from build123d import *

# Parameters (mm, degrees)
SKETCH1_W           = 26
SKETCH1_H           = 10
BOSS_EXTRUDE1_DEPTH = 4


with BuildPart() as part:
    # Sketch1 → Boss-Extrude1 (new body)
    with BuildSketch(Plane.XY):
        with Locations((13, 5)):
            Rectangle(SKETCH1_W, SKETCH1_H)
        Polygon((2.899999851, 6.905256103), (4.382026, 7.166577107), (5.68529807, 6.414133033), (6.200000003, 5.000000051), (5.68529807, 3.585867069), (4.382026, 2.833422995), (2.899999851, 3.094743999), (1.932676008, 4.247555672), (1.932676008, 5.75244443), align=None, mode=Mode.SUBTRACT)
        Polygon((20.899999848, 6.905256103), (22.382025996, 7.166577107), (23.685298066, 6.414133033), (24.2, 5.000000051), (23.685298066, 3.585867069), (22.382025996, 2.833422995), (20.899999848, 3.094743999), (19.932676005, 4.247555672), (19.932676005, 5.75244443), align=None, mode=Mode.SUBTRACT)
    extrude(amount=BOSS_EXTRUDE1_DEPTH)


solid = part.part
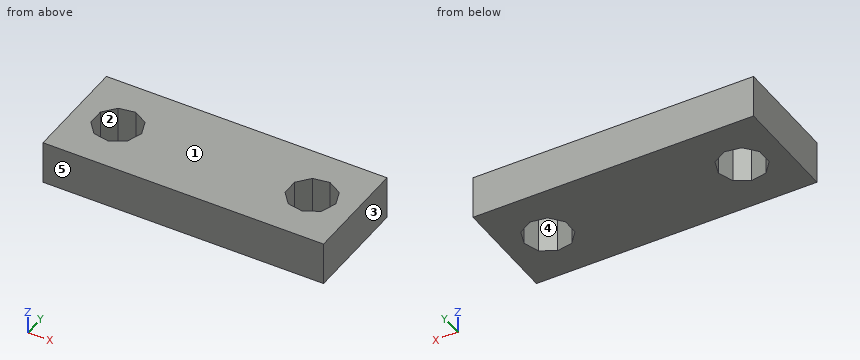
For this review, take the finished solid that the model builds, in its own axes (mm). Face numbers are marked on the shaded views. A direction names the side the tool comes from. Give positions to 0.01 mm unless a question says otherwise; leave off trailing zeros. Loops run counter-clockwise (first coordinate to the right, second up) from the corner with the lowest first, then second, coordinate; pieces in that order, holes last.
Item 1: Take a section at B-B, the plane x = 22.75. State the section outline as (y, z) points.
Item 2: Take a section at A-A, the plane z = 1.25. State the section outline as (x, y) points, and give its area (3 significant figures).
Item 3: Draft analysis for pull direction X (two halves, no side actions). For the marked faces 1, 2 and 3, state which applies: +X half, -X half, draft (parallel to the pull), parting line (faces both ways), or undercut.
Item 4: Tool access review of the marked faces 4 and 5: name each direction out of +Z, -Z, +X, -X, +Y, -Y from which nothing blocks a thin tool from reaching the whole face with its end or side.
Item 5: For line 1 along X through (y, z) = (3.5, 2.6); line 2 along Y through (x, z) = (4.75, 3.4); line 3 along X through (y, z) = (5.75, 1.6), list the stretches that pass through material, from the lowest coordinate up.
Item 6: Insertion check: pin 1 (2 mm diameter, centred on y = 3, z = 3, fed in from -X). The pin has a flat end and moves straight along its axis. Give the tip position at first contact, or say it passes through.
Calculated:
1. outline: (0, 0) - (3.05, 0) - (3.05, 4) - (0, 4) - close; (6.95, 0) - (10, 0) - (10, 4) - (6.95, 4) - close
2. outline: (0, 0) - (26, 0) - (26, 10) - (0, 10) - close; hole (1.93, 4.25) - (2.9, 3.09) - (4.38, 2.83) - (5.69, 3.59) - (6.2, 5) - (5.69, 6.41) - (4.38, 7.17) - (2.9, 6.91) - (1.93, 5.75) - close; hole (19.93, 4.25) - (20.9, 3.09) - (22.38, 2.83) - (23.69, 3.59) - (24.2, 5) - (23.69, 6.41) - (22.38, 7.17) - (20.9, 6.91) - (19.93, 5.75) - close
2. area: 232 mm2
3. face 1: draft
3. face 2: undercut
3. face 3: +X half
4. face 4: +Z, -Z
4. face 5: +Z, -Z, +X, -X, -Y
5. line 1: x = 0 to 2.56, 5.54 to 20.56, 23.54 to 26
5. line 2: y = 0 to 3.05, 6.95 to 10
5. line 3: x = 0 to 1.93, 5.93 to 19.93, 23.93 to 26
6. pin 1: stops at x = 0
